Part model, mm, in its own coordinate system. Face numbers are marked on the shaded views. A direction names the side the tool comes from. Coordinates: 2 decimals unless noted, no trailing zeros. Loops run counter-clockwise (first coordinate to the right, second up) from the corner with the lowest first, then second, coordinate; pieces in that order, holes last. Notation, with made-up numbers: (11.5, 75) -> (26.5, 75) arc R28 cw to (26.5, 109) -> close; hole circle Ø3 at (-14.75, 48). An arc over 180 degrees is marked (long way). One line per question, with ' | ' between items. Start each with the question number.
1) Drop flat-ended pins along their axis: pin 1 (5 mm diameter, centred on y = 11.5, z = 10, fed in from +X); pin 2 (5 mm diameter, centred on x = 29, z = 9, fed in from +Y); pin 3 (1.9 mm diameter, centred on x = 5, z = 7.5, fed in from +Y); pin 4 (8 mm diameter, centred on y = 7, z = 5, fed in from -X). Give the stop position or say it passes through.
2) Probe L1, parallel to X at y = 9, z = 11.7; L2, parallel to Z at x = 5, y = 1; L3, parallel to X at y = 9, z = 4.25. List the from-to ranges inside material, lowest first. Write a range as from..to.
3) Cut at A-A (y = 9). List the corners of the cut face in (x, z), plus the area to 3 significant figures.
4) Cut at B-B (x = 17). List the corners of the cut face in (y, z).
5) Cut at D-D (x = 29). List the corners of the cut face in (y, z).
6) Two-plate mould, pull along X, no slides. Class the marked faces 1, 2 and 3: released by +X, released by -X, zero draft, split by the parting line, or undercut.
7) Cut at C-C (y = 1.25). List the corners of the cut face in (x, z), plus the area to 3 significant figures.
8) 3-axis set-ups, long thin cutter, end or side, ignore diameter. For the marked faces 4 and 5: which of +Z, -Z, +X, -X, +Y, -Y reach the whole face in a straight line?
from build123d import *

# Parameters (mm, degrees)
SKETCH_R        = 2
PAD_DEPTH       = 15
SKETCH001_R     = 4.7
POCKET_DEPTH    = 10
SKETCH002_R     = 1.6
POCKET001_DEPTH = 2.001
FILLET_R        = 2
FILLET001_R     = 3
FILLET002_R     = 1


with BuildPart() as part:
    # Sketch → Pad (new body)
    with BuildSketch(Plane.XY):
        Polygon((0, 0), (34, 0), (34, 2), (24, 2), (24, 16), (10, 16), (10, 2), (0, 2), align=None)
        with Locations((17, 9)):
            Circle(SKETCH_R, mode=Mode.SUBTRACT)
    extrude(amount=PAD_DEPTH)

    # Sketch001 (on Face10 of Pad) → Pocket (cut)
    with BuildSketch(Plane(origin=(0, 0, 0), x_dir=(1, 0, 0), z_dir=(0, 0, -1))):
        with Locations((17, -9)):
            Circle(SKETCH001_R)
    extrude(amount=-POCKET_DEPTH, mode=Mode.SUBTRACT)

    # Sketch002 (on Face7 of Pocket) → Pocket001 (cut, through all)
    with BuildSketch(Plane(origin=(0, 2, 0), x_dir=(-1, 0, 0), z_dir=(0, 1, 0))):
        with Locations((-29, 7.5)):
            Circle(SKETCH002_R)
        with Locations((-5, 7.5)):
            Circle(SKETCH002_R)
    extrude(amount=-POCKET001_DEPTH, mode=Mode.SUBTRACT)

    # Fillet
    fillet_edges = [part.edges().sort_by_distance(p)[0] for p in [
        (34, 1, 15),
        (34, 1, 0),
        (0, 1, 15),
        (0, 1, 0),
    ]]
    fillet(fillet_edges, radius=FILLET_R)

    # Fillet001
    fillet001_edges = [part.edges().sort_by_distance(p)[0] for p in [
        (24, 16, 7.5),
        (10, 16, 7.5),
    ]]
    fillet(fillet001_edges, radius=FILLET001_R)

    # Fillet002
    fillet002_edges = [part.edges().sort_by_distance(p)[0] for p in [
        (24, 2, 7.5),
        (10, 2, 7.5),
    ]]
    fillet(fillet002_edges, radius=FILLET002_R)


solid = part.part
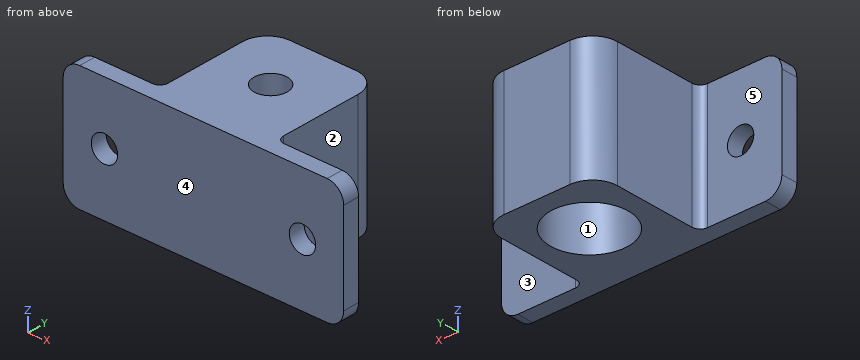
Reported:
1) pin 1: stops at x = 24 | pin 2: stops at y = 2 | pin 3: passes through | pin 4: stops at x = 10
2) L1: x = 10..15, 19..24 | L2: z = 0..5.9, 9.1..15 | L3: x = 10..12.3, 21.7..24
3) outline: (10, 0) -> (12.3, 0) -> (12.3, 10) -> (15, 10) -> (15, 15) -> (10, 15) -> close; (19, 10) -> (21.7, 10) -> (21.7, 0) -> (24, 0) -> (24, 15) -> (19, 15) -> close | area: 96.0 mm²
4) outline: (0, 0) -> (4.3, 0) -> (4.3, 10) -> (7, 10) -> (7, 15) -> (0, 15) -> close; (11, 10) -> (13.7, 10) -> (13.7, 0) -> (16, 0) -> (16, 15) -> (11, 15) -> close
5) outline: (0, 0) -> (2, 0) -> (2, 5.9) -> (0, 5.9) -> close; (0, 9.1) -> (2, 9.1) -> (2, 15) -> (0, 15) -> close
6) face 1: undercut | face 2: released by +X | face 3: zero draft
7) outline: (0, 2) arc R2 ccw to (2, 0) -> (32, 0) arc R2 ccw to (34, 2) -> (34, 13) arc R2 ccw to (32, 15) -> (2, 15) arc R2 ccw to (0, 13) -> close; hole circle Ø3.2 at (5, 7.5); hole circle Ø3.2 at (29, 7.5) | area: 490 mm²
8) face 4: +Z, -Z, +X, -X, -Y | face 5: +Z, -Z, -X, +Y
